Work out the finished part from the listing and answer in its coordinate system (mm). Face numbers are marked on the shaded views. Give positions to 0.01 mm unless a question says otherwise; leave off trailing zeros. Write each loop counter-clockwise with the first axis right and the second up, starting at its lowest first coordinate (ties: lowest second). Pieces come first, ordered by that corner, then holes.
1) Given pin 1 Ø2 at (x, z) = (16, 19) entering from +Y; pin 2 Ø1.5 at (x, z) = (-24.5, 13.5) entering from +Y; pin 3 Ø6.5 at (x, y) = (17.32, -10) entering from +Z, each flat-ended and moving along its own axis, determine where each tip first touches the part or whether it passes through.
2) Find section C-C (y = 0). Determine the outline of the cut face in (x, z), plus the area to 3 significant figures.
3) Straight lines are drawn through the part: probe 1 along Y at (x, z) = (0, 20.5); probe 2 along Y at (x, z) = (0, 8); probe 3 along Z at (x, y) = (-12, -11.5). For each, find the intervals that lie inside material, in ascending order.
4) Find section B-B (z = 21). Determine the outline of the cut face in (x, y), plus the area to 3 significant figures.
5) Find section D-D (y = -10). Count the separate pieces of the cut face and the enclosed holes in it, plus the area to 3 significant figures.
6) Find section A-A (x = 0). Determine the outline of the cut face in (y, z), plus the area to 3 significant figures.
7) Determine the mould class of the marked faces 1, 2 and 3 for opening direction Y: pulls with the +Y half, pulls with the -Y half, needs draft (parallel to the pull), parting line crosses it, or undercut.
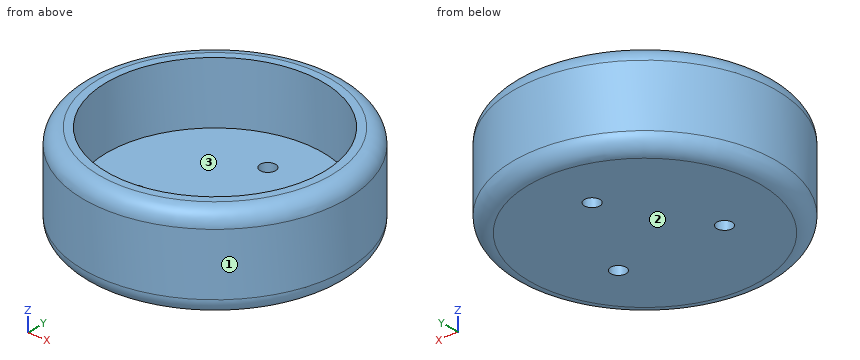
```python
from build123d import *

# Parameters (mm, degrees)
SKETCH2_R           = 42.5
BOSS_EXTRUDE2_DEPTH = 30
SKETCH3_OUTSIDE_W   = 111.78
SKETCH3_OUTSIDE_H   = 111.78
SKETCH3_OUTSIDE_R   = 42.5
SKETCH3_OUTSIDE_R_2 = 35
CUT_EXTRUDE2_DEPTH  = 20
SKETCH8_R           = 2.5
CUT_EXTRUDE3_DEPTH  = 10
FILLET3_R           = 5


with BuildPart() as part:
    # Sketch2 → Boss-Extrude2 (new body)
    with BuildSketch(Plane.XY):
        Circle(SKETCH2_R)
    extrude(amount=BOSS_EXTRUDE2_DEPTH)

    # Sketch3 outside → Cut-Extrude2 (cut)
    # profile 1 of 2: a face of its own
    with BuildSketch(Plane.XY.offset(30)):
        Rectangle(SKETCH3_OUTSIDE_W, SKETCH3_OUTSIDE_H)
        Circle(SKETCH3_OUTSIDE_R, mode=Mode.SUBTRACT)
    # profile 2 of 2: a face of its own
    with BuildSketch(Plane.XY.offset(30)):
        Circle(SKETCH3_OUTSIDE_R_2)
    extrude(amount=-CUT_EXTRUDE2_DEPTH, mode=Mode.SUBTRACT)

    # Sketch8 → Cut-Extrude3 (cut)
    with BuildSketch(Plane.XY.offset(10)):
        with Locations((0, 20)):
            Circle(SKETCH8_R)
        with Locations((17.320508076, -10)):
            Circle(SKETCH8_R)
        with Locations((-17.320508076, -10)):
            Circle(SKETCH8_R)
    extrude(amount=-CUT_EXTRUDE3_DEPTH, mode=Mode.SUBTRACT)

    # Fillet3
    fillet3_edges = [part.edges().sort_by_distance(p)[0] for p in [
        (-42.5, 0, 0),
        (-42.5, 0, 30),
    ]]
    fillet(fillet3_edges, radius=FILLET3_R)


solid = part.part
```
Results:
1. pin 1: stops at y = 39.76
1. pin 2: stops at y = 35.24
1. pin 3: stops at z = 10
2. outline: (-42.5, 5) arc R5 ccw to (-37.5, 0) - (37.5, 0) arc R5 ccw to (42.5, 5) - (42.5, 25) arc R5 ccw to (37.5, 30) - (35, 30) - (35, 10) - (-35, 10) - (-35, 30) - (-37.5, 30) arc R5 ccw to (-42.5, 25) - close
2. area: 1,130 mm2
3. probe 1: y = -42.5 to -35, 35 to 42.5
3. probe 2: y = -42.5 to 17.5, 22.5 to 42.5
3. probe 3: z = 0 to 10
4. outline: circle Ø85 at (0, 0); hole circle Ø70 at (0, 0)
4. area: 1,830 mm2
5. separate pieces: 3
5. enclosed holes: 0
5. area: 1,010 mm2
6. outline: (-42.5, 5) arc R5 ccw to (-37.5, 0) - (17.5, 0) - (17.5, 10) - (-35, 10) - (-35, 30) - (-37.5, 30) arc R5 ccw to (-42.5, 25) - close; (22.5, 0) - (37.5, 0) arc R5 ccw to (42.5, 5) - (42.5, 25) arc R5 ccw to (37.5, 30) - (35, 30) - (35, 10) - (22.5, 10) - close
6. area: 1,080 mm2
7. face 1: parting line crosses it
7. face 2: needs draft
7. face 3: undercut
